Check sheet for the modelled part. Datum: model origin and axes. Units: mm. Coordinates: 2 decimals unless noted, no trailing zeros. Loops run counter-clockwise (first coordinate to the right, second up) from the corner with the lowest first, then second, coordinate; pieces in that order, holes last. Notation, with made-up numbers: (-6.75, 54.25) - (-2.75, 54.25) arc R16 cw to (-2.75, 70.25) - close; hole circle Ø6 at (-29, 20). An arc over 180 degrees is marked (long way). Use a Markdown table: item, result. Add a question column.
1) Draft check along Z on faces 1 (the cylindrical face through (-0.434, -1.952, 7.746)), 2 (the flat face through (0, 0, 8.5)), 3 (the cylindrical face through (-1.5, 0.07, 3.7)). Enter one of: pulls with the +Z half, pulls with the -Z half, needs draft (parallel to the pull), parting line crosses it, or undercut.
2) Sectioned sample at A-A, the plane x = 0. Enter the section's corners in (y, z), then the cut area to 3 significant figures.
3) Thickness scan on line 1 (X direction, y = -0.05, z = 1); line 2 (Z direction, x = 1.6, y = 1); line 3 (X direction, y = 1.05, z = 0.5). Record the ranges inside material, lowest first.
4) Sectioned sample at C-C, the plane z = 2.5. Enter the section's corners in (x, y), then the cut area to 3 significant figures.
5) Go/stop test with flat-tipped pins: P1, Ø1, axis at y = -0.5, z = 2, coming from the +X side; P2, Ø1.5, axis at x = 0.5, z = 1, coming from the -Y side. Record where each tip stops, or that it passes through.
from build123d import *

# Parameters (mm, degrees)
SKETCH1_R           = 1.5
BOSS_EXTRUDE1_DEPTH = 7.5
SKETCH2_R           = 2
BOSS_EXTRUDE2_DEPTH = 1
SKETCH3_R           = 2
BOSS_EXTRUDE3_DEPTH = 1
FILLET1_R           = 0.5


with BuildPart() as part:
    # Sketch1 → Boss-Extrude1 (new body)
    with BuildSketch(Plane.XY):
        Circle(SKETCH1_R)
    extrude(amount=BOSS_EXTRUDE1_DEPTH)

    # Sketch2 → Boss-Extrude2 (add)
    with BuildSketch(Plane(origin=(0, 0, 0), x_dir=(-1, 0, 0), z_dir=(0, 0, -1))):
        Circle(SKETCH2_R)
    extrude(amount=BOSS_EXTRUDE2_DEPTH)

    # Sketch3 → Boss-Extrude3 (add)
    with BuildSketch(Plane.XY.offset(7.5)):
        Circle(SKETCH3_R)
    extrude(amount=BOSS_EXTRUDE3_DEPTH)

    # Fillet1
    fillet1_edges = [part.edges().sort_by_distance(p)[0] for p in [
        (-2, 0, 8.5),
        (2, 0, -1),
    ]]
    fillet(fillet1_edges, radius=FILLET1_R)


solid = part.part
Solved:
| question | item | result |
|---|---|---|
| 1 | face 1 | needs draft |
| 1 | face 2 | pulls with the +Z half |
| 1 | face 3 | undercut |
| 2 | outline | (-2, -0.5) arc R0.5 ccw to (-1.5, -1) - (1.5, -1) arc R0.5 ccw to (2, -0.5) - (2, 0) - (1.5, 0) - (1.5, 7.5) - (2, 7.5) - (2, 8) arc R0.5 ccw to (1.5, 8.5) - (-1.5, 8.5) arc R0.5 ccw to (-2, 8) - (-2, 7.5) - (-1.5, 7.5) - (-1.5, 0) - (-2, 0) - close |
| 2 | area | 30.3 mm2 |
| 3 | line 1 | x = -1.5 to 1.5 |
| 3 | line 2 | z = -0.82 to 0, 7.5 to 8.32 |
| 3 | line 3 | x = -1.07 to 1.07 |
| 4 | outline | circle Ø3 at (0, 0) |
| 4 | area | 7.07 mm2 |
| 5 | P1 | stops at x = 1.5 |
| 5 | P2 | stops at y = -1.5 |
